Geometry check sheet. Reference: the model listing, model coordinates, mm. Give positions to 0.01 mm unless a question says otherwise; leave off trailing zeros. Order: outer loops, then holes, each group sorted by start corner. A loop starts at its lowest first (then second) coordinate and runs counter-clockwise, first axis right, second up. Notation, with made-up numbers: M -16,87 L 27,87 A19 cw 27,92 Z; hole C 2,58.25 d11. An arc over 180 degrees is marked long. Answer as CSV lines item,"result". Start each with the question number.
Q1. Section check C-C, the plane z = 4.5. Record the boundary of the cut face in (x, y), then the cut area to 3 significant figures.
Q2. Section check D-D, the plane z = 19.5. Record the boundary of the cut face in (x, y).
Q3. Section check B-B, the plane y = -1.65. Record the boundary of the cut face in (x, z) (1 decimal).
Q4. Go/stop test with flat-tipped pins: pin 1 (1.5 mm diameter, centred on y = -1, z = 18, fed in from +X); pin 2 (1.3 mm diameter, centred on x = 4, y = -1, fed in from -Z); pin 3 (1 mm diameter, centred on y = -1.5, z = 17, fed in from +X). Record where each tip stops, or that it passes through.
Q5. Thickness scan on line 1 (X direction, y = -2.75, z = 0) (3 decimals); line 2 (X direction, y = -0.7, z = 1) (3 decimals); line 3 (X direction, y = -1.45, z = 38.5). Record the ranges inside material, lowest first.
Q6. Section check A-A, the plane x = 0. Record the boundary of the cut face in (y, z).
```python
from build123d import *

# Parameters (mm, degrees)
F1_DEPTH = 3
F2_R     = 1
F3_R     = 1
F4_R     = 1


with BuildPart() as f1:
    # F0 (on Front) → F1 (new body)
    with BuildSketch(Plane.XZ):
        with BuildLine():
            ThreePointArc((-2, 5.0159744816), (-3.0298514815, -4.4698993277), (5.4, 0))
            ThreePointArc((5.4, 0), (4.4698993277, 3.0298514815), (2, 5.0159744816))
            Line((2, 5.0159744816), (0, 5.0159744816))
            Line((0, 5.0159744816), (-2, 5.0159744816))
        make_face()
        with BuildLine():
            ThreePointArc((1.525, 2.1057955741), (2.3157072354, 1.1821590418), (2.6, 0))
            ThreePointArc((2.6, 0), (2.3157072354, -1.1821590418), (1.525, -2.1057955741))
            ThreePointArc((1.525, -2.1057955741), (0, -2.6), (-1.525, -2.1057955741))
            ThreePointArc((-1.525, -2.1057955741), (-2.6, 0), (-1.525, 2.1057955741))
            ThreePointArc((-1.525, 2.1057955741), (0, 2.6), (1.525, 2.1057955741))
        make_face(mode=Mode.SUBTRACT)
        with BuildLine():
            Line((0, 5.0159744816), (2, 5.0159744816))
            ThreePointArc((2, 5.0159744816), (0, 5.4), (-2, 5.0159744816))
            Line((-2, 5.0159744816), (0, 5.0159744816))
        make_face()
        with BuildLine():
            ThreePointArc((-2, 5.0159744816), (0, 5.4), (2, 5.0159744816))
            Line((2, 5.0159744816), (3.0470652436, 35))
            Line((3.0470652436, 35), (0, 35))
            Line((0, 35), (-3.0470652436, 35))
            Line((-3.0470652436, 35), (-2, 5.0159744816))
        make_face()
        Polygon((0, 35), (3.0470652436, 35), (7.5, 35), (0, 47.5), (-7.5, 35), (-3.0470652436, 35), align=None)
        with BuildLine():
            ThreePointArc((1.525, -2.1057955741), (2.3157072354, -1.1821590418), (2.6, 0))
            ThreePointArc((2.6, 0), (2.3157072354, 1.1821590418), (1.525, 2.1057955741))
            Line((1.525, 2.1057955741), (1.525, -2.1057955741))
        make_face()
        with BuildLine():
            Line((-1.525, -2.1057955741), (-1.525, 2.1057955741))
            ThreePointArc((-1.525, 2.1057955741), (-2.6, 0), (-1.525, -2.1057955741))
        make_face()
    extrude(amount=F1_DEPTH)

    # F2
    f2_edges = [f1.edges().sort_by_distance(p)[0] for p in [
        (0, -1.5, 47.5),
    ]]
    fillet(f2_edges, radius=F2_R)

    # F3
    f3_edges = [f1.edges().sort_by_distance(p)[0] for p in [
        (-7.5, -1.5, 35),
    ]]
    fillet(f3_edges, radius=F3_R)

    # F4
    f4_edges = [f1.edges().sort_by_distance(p)[0] for p in [
        (7.5, -1.5, 35),
    ]]
    fillet(f4_edges, radius=F4_R)


solid = f1.part
```
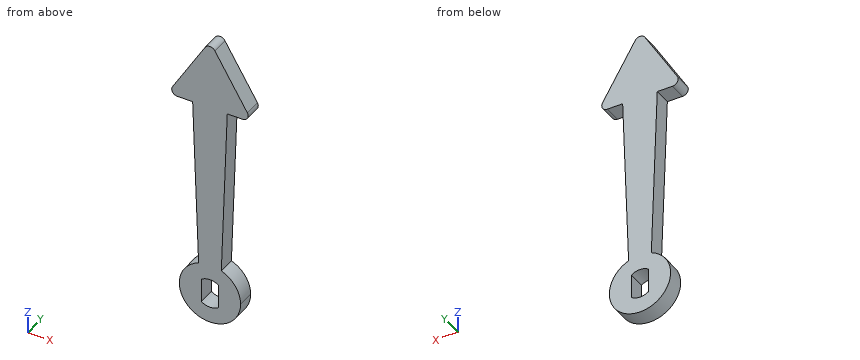
Answer block:
1,outline,"M -2.98,-3 L 2.98,-3 L 2.98,0 L -2.98,0 Z"
1,area,"17.9 mm2"
2,outline,"M -2.51,-3 L 2.51,-3 L 2.51,0 L -2.51,0 Z"
3,outline,"M -6.6,36.5 A1 ccw -5.7,35 L -3,35 L -2,5 A5.4 ccw long 2,5 L 3,35 L 5.7,35 A1 ccw 6.6,36.5 L 0.9,46.1 A1 ccw -0.9,46.1 Z; hole M -1.5,-2.1 A2.6 ccw 1.5,-2.1 L 1.5,2.1 A2.6 ccw -1.5,2.1 Z"
4,pin 1,"stops at x = 2.48"
4,pin 2,"stops at z = -4.24"
4,pin 3,"stops at x = 2.44"
5,line 1,"x = -5.4 to -1.525, 1.525 to 5.4"
5,line 2,"x = -5.307 to -1.525, 1.525 to 5.307"
5,line 3,"x = -5.4 to 5.4"
6,outline,"M -3,-5.4 L 0,-5.4 L 0,-2.6 L -3,-2.6 Z; M -3,2.6 L 0,2.6 L 0,46.56 L -3,46.56 Z"
